```python
from build123d import *

# Parameters (mm, degrees)
SKETCH_1_R      = 1.6
EXTRUDE_1_DEPTH = 1.5
SKETCH_2_W      = 29.5
SKETCH_2_H      = 3.75
SKETCH_2_H_2    = 2.75
EXTRUDE_2_DEPTH = 7.2
SKETCH_3_W      = 29.5
SKETCH_3_H      = 8.4
EXTRUDE_3_DEPTH = 6.3


with BuildPart() as part:
    # ｽｹｯﾁ1 → ﾎﾞｽ - 押し出し1 (new body)
    with BuildSketch(Plane.XY):
        with BuildLine():
            Line((0, 3.75), (37, 3.75))
            ThreePointArc((37, 3.75), (40.75, 0), (37, -3.75))
            Line((37, -3.75), (0, -3.75))
            ThreePointArc((0, -3.75), (-3.75, 0), (0, 3.75))
        make_face()
        Circle(SKETCH_1_R, mode=Mode.SUBTRACT)
        with Locations((37, 0)):
            Circle(SKETCH_1_R, mode=Mode.SUBTRACT)
    extrude(amount=EXTRUDE_1_DEPTH)

    # ｽｹｯﾁ2 → ﾎﾞｽ - 押し出し2 (add)
    with BuildSketch(Plane(origin=(0, 0, 0), x_dir=(-1, 0, 0), z_dir=(0, 0, -1))):
        with Locations((-18.5, -1.875)):
            Rectangle(SKETCH_2_W, SKETCH_2_H)
        with Locations((-18.5, 1.875)):
            Rectangle(SKETCH_2_W, SKETCH_2_H)
        with Locations((-18.5, 5.125)):
            Rectangle(SKETCH_2_W, SKETCH_2_H_2)
        with Locations((-18.5, -5.125)):
            Rectangle(SKETCH_2_W, SKETCH_2_H_2)
    extrude(amount=-EXTRUDE_2_DEPTH)

    # ｽｹｯﾁ3 → ﾎﾞｽ - 押し出し3 (add)
    with BuildSketch(Plane.XY.offset(7.2)):
        with Locations((18.5, 0)):
            Rectangle(SKETCH_3_W, SKETCH_3_H)
    extrude(amount=EXTRUDE_3_DEPTH)


solid = part.part
```
Source: CAD feature listing. Evaluate the final solid. Frame: model axes, mm. A direction names the side the tool comes from. Coordinates: 2 decimals unless noted, no trailing zeros. Loops run counter-clockwise (first coordinate to the right, second up) from the corner with the lowest first, then second, coordinate; pieces in that order, holes last. Notation, with made-up numbers: M 82.5,-0.5 L 118.5,-0.5 A29 cw 118.5,20.5 Z; hole C 37,71 d2. An arc over 180 degrees is marked long. Use CSV: the item, a comma, the result in double quotes.
(1) Cut plane B-B on x = 5. Return loops of the section in (y, z), and give its area (3 significant figures).
Answers follow:
outline,"M -6.5,0 L 6.5,0 L 6.5,7.2 L 4.2,7.2 L 4.2,13.5 L -4.2,13.5 L -4.2,7.2 L -6.5,7.2 Z"
area,"147 mm²"
(2) Cut plane C-C on y = -3. Return loops of the section in (x, z), and give its area (3 significant figures).
Answers follow:
outline,"M -2.25,0 L 39.25,0 L 39.25,1.5 L 33.25,1.5 L 33.25,13.5 L 3.75,13.5 L 3.75,1.5 L -2.25,1.5 Z"
area,"416 mm²"
(3) Draft query along Y for faces 4 (the face through (-3.75, -0.08, 0.74)), 5 (the face through (-1.27, -0.97, 0.74)), 6 (the face through (19, 5, 7.2)), 7 (the face through (35.82, 1.08, 0.74)). Return one class per face: pulls with the +Y half, pulls with the -Y half, needs draft (parallel to the pull), parting line crosses it, or undercut.
Answers follow:
face 4,"parting line crosses it"
face 5,"undercut"
face 6,"needs draft"
face 7,"undercut"
(4) Cut plane A-A on y = 0. Return loops of the section in (x, z).
Answers follow:
outline,"M -3.75,0 L -1.6,0 L -1.6,1.5 L -3.75,1.5 Z; M 1.6,0 L 35.4,0 L 35.4,1.5 L 33.25,1.5 L 33.25,13.5 L 3.75,13.5 L 3.75,1.5 L 1.6,1.5 Z; M 38.6,0 L 40.75,0 L 40.75,1.5 L 38.6,1.5 Z"
(5) Cut plane D-D on z = 9.75. Return loops of the section in (x, y), and give its area (3 significant figures).
Answers follow:
outline,"M 3.75,-4.2 L 33.25,-4.2 L 33.25,4.2 L 3.75,4.2 Z"
area,"248 mm²"
(6) Line query: line 1 (Y direction, x = 37, z = 1.05); line 2 (Z direction, x = 30, y = 5.5). Output: solid intervals per line, ascending. Write a range as [from, to].
Answers follow:
line 1,"[-3.75, -1.6], [1.6, 3.75]"
line 2,"[0, 7.2]"
(7) Contact query for flat-ended pins moving along their axis: pin 1 (1.6 mm diameter, centred on x = 34.5, z = 0.5, fed in from +Y); pin 2 (1.2 mm diameter, centred on x = 16.5, y = -5.5, fed in from +Z); pin 3 (5 mm diameter, centred on x = 0, y = 0, fed in from +Z). Output: stop coordinate, or through.
Answers follow:
pin 1,"y = 3.75"
pin 2,"z = 7.2"
pin 3,"z = 1.5"
(8) Reachability of faces 1 (the face through (2, -3.75, 1)), 2 (the face through (19, -5, 7.2)), 3 (the face through (2, 3.75, 1)) from +Z, -Z, +X, -X, +Y, -Y: full face, straight path, thin tool, end or side. Return the list, or none.
Answers follow:
face 1,"+Z, -Z, -X, -Y"
face 2,"+Z, +X, -X, -Y"
face 3,"+Z, -Z, -X, +Y"
